Design review of the part built by this model. Coordinates are the model's own, in mm. A direction names the side the tool comes from. Coordinates: 2 decimals unless noted, no trailing zeros. Loops run counter-clockwise (first coordinate to the right, second up) from the corner with the lowest first, then second, coordinate; pieces in that order, holes last.
Q1. Add section A-A on z = 1.5. Give the boundary of the cut face in (x, y), and give its area (3 significant figures).
Q2. Add section B-B on x = -42. Give the boundary of the cut face in (y, z) (1 decimal), and give its area (3 significant figures).
Q3. Add section D-D on x = -24. Give the boundary of the cut face in (y, z).
Q4. Add section C-C on y = 926.5. Give the boundary of the cut face in (x, z) (1 decimal), and give its area (3 significant figures).
Q5. Machinability: for faces 4 (the face through (-40, 831.5, 2)), 5 (the face through (-41.302, 936.415, -3.072)), 6 (the face through (-25.54, 843.94, 4.31)), which of the approach directions +Z, -Z, +X, -X, +Y, -Y give a long, thin tool a straight path to every point of the face, cutting with its end or side? Answer none if there is none.
Q6. Draft analysis for pull direction X (two halves, no side actions). For faces 1 (the face through (-61.99, 834.35, 1.68)), 2 (the face through (-40, 887, 0)), 3 (the face through (-55.54, 843.94, 4.31)), state which applies: released by +X, released by -X, zero draft, split by the parting line, or undercut.
Q7. For P1, Ø10, axis at x = -34.5, y = 901.5, coming from the -Z side; P2, Ø2.5, axis at x = -54, y = 840.5, coming from the +Z side; P3, Ø12, axis at x = -42.5, y = 883.5, coming from the +Z side, all flat-tipped, find the tip position at first contact; note any pin that passes through.
Q8. Wall thickness on probe 1 along Z at (x, y) = (-28, 855.5); probe 2 along Y at (x, z) = (-34, 2.5); probe 3 along Y at (x, z) = (-52, 1.25): over which ranges is each line inside the solid? List them lowest first.
Autodesk Inventor part; units mm, degrees
ref_plane "YZ Plane" through (0, 0, 0) normal (1, 0, 0) x (0, 1, 0)
ref_plane "XZ Plane" through (0, 0, 0) normal (0, 1, 0) x (-1, 0, 0)
ref_plane "XY Plane" through (0, 0, 0) normal (0, 0, 1) x (1, 0, 0)
sketch "Sketch1" plane through (0, 0, 0) normal (0, 0, 1) x (1, 0, 0)
  circle A0 centre (-40, 926.5) radius 10
  circle A1 centre (-40, 926.5) radius 14
  line L0 (-65, 921.2927) -> (-65, 841.5)
  line L1 (-55, 831.5) -> (-40, 831.5)
  arc A2 (-60, 929.953) -> (-65, 921.2927) centre (-55, 921.2927) ccw
  arc A3 (-65, 841.5) -> (-55, 831.5) centre (-55, 841.5) ccw
  line L2 (-40, 926.5) -> (-40, 831.5) construction
  line L3 (-40, 936.5) -> (-40, 831.5) construction
  circle A4 centre (-40, 926.5) radius 10
  line L4 (-15, 921.2927) -> (-15, 841.5)
  line L5 (-25, 831.5) -> (-40, 831.5)
  arc A5 (-15, 921.2927) -> (-20, 929.953) centre (-25, 921.2927) ccw
  arc A6 (-25, 831.5) -> (-15, 841.5) centre (-25, 841.5) ccw
  line L6 (-60, 929.953) -> (-43.2258, 939.6376)
  line L7 (-36.7742, 939.6376) -> (-20, 929.953)
  arc A7 (-36.7742, 939.6376) -> (-43.2258, 939.6376) centre (-40, 934.0503) ccw
  point P0 (0, 0)
  point P1 (-40, 941.5)
  dimension "d0" = 10
  dimension "d1" = 25
  dimension "d3" = 95
  dimension "d4" = 15
  dimension "d5" = 6.4516
  dimension "d6" = 120
  dimension "d7" = 4.3301
extrude "Extrusion1" add sketch "Sketch1" along normal blind 3.4125 contours A0 | A1 L6 A7 L7 | A1 L7 A5 L4 A6 L5 L1 A3 L0 A2 L6
sketch "Sketch2" plane through (0, 0, 3.4125) normal (0, 0, 1) x (1, 0, 0)
  circle A0 centre (-40, 926.5) radius 10
  circle A1 centre (-40, 926.5) radius 10
  point P0 (0, 0)
extrude "Extrusion2" add sketch "Sketch2" along normal blind 3.4125 and the other way blind 9.6435
sketch "Sketch3" plane through (-40, 926.5, 6.825) normal (0, 0, 1) x (1, 0, 0)
  circle A0 centre (0, 0) radius 10
  point P0 (40, -926.5)
sketch "Sketch4" plane through (0, 0, 3.4125) normal (0, 0, 1) x (1, 0, 0)
  arc A0 (-65, 841.5) -> (-55, 831.5) centre (-55, 841.5) ccw
  arc A1 (-25, 831.5) -> (-15, 841.5) centre (-25, 841.5) ccw
  circle A2 centre (-55, 841.5) radius 2.5
  circle A3 centre (-25, 841.5) radius 2.5
  point P0 (0, 0)
  dimension "d14" = 5
extrude "Extrusion3" add sketch "Sketch4" along normal blind 1.825
properties part number "WheelHolder"
Entries:
1. outline: (-65, 841.5) arc R10 ccw to (-55, 831.5) - (-25, 831.5) arc R10 ccw to (-15, 841.5) - (-15, 921.29) arc R10 ccw to (-20, 929.95) - (-36.77, 939.64) arc R6.45 ccw to (-43.23, 939.64) - (-60, 929.95) arc R10 ccw to (-65, 921.29) - close
1. area: 5,080 mm2
2. outline: (831.5, 0) - (916.7, 0) - (916.7, -6.2) - (936.3, -6.2) - (936.3, 0) - (940.2, 0) - (940.2, 3.4) - (936.3, 3.4) - (936.3, 6.8) - (916.7, 6.8) - (916.7, 3.4) - (831.5, 3.4) - close
2. area: 560 mm2
3. outline: (831.55, 0) - (932.26, 0) - (932.26, 3.41) - (843.79, 3.41) - (843.79, 5.24) - (839.21, 5.24) - (839.21, 3.41) - (831.55, 3.41) - close
4. outline: (-63.5, 0) - (-50, 0) - (-50, -6.2) - (-30, -6.2) - (-30, 0) - (-16.5, 0) - (-16.5, 3.4) - (-30, 3.4) - (-30, 6.8) - (-50, 6.8) - (-50, 3.4) - (-63.5, 3.4) - close
4. area: 354 mm2
5. face 4: +Z, -Z, +X, -X, -Y
5. face 5: -Z
5. face 6: +Z
6. face 1: released by -X
6. face 2: zero draft
6. face 3: undercut
7. P1: stops at z = 0
7. P2: stops at z = 5.24
7. P3: stops at z = 3.41
8. probe 1: z = 0 to 3.41
8. probe 2: y = 831.5 to 938.04
8. probe 3: y = 831.5 to 934.57
